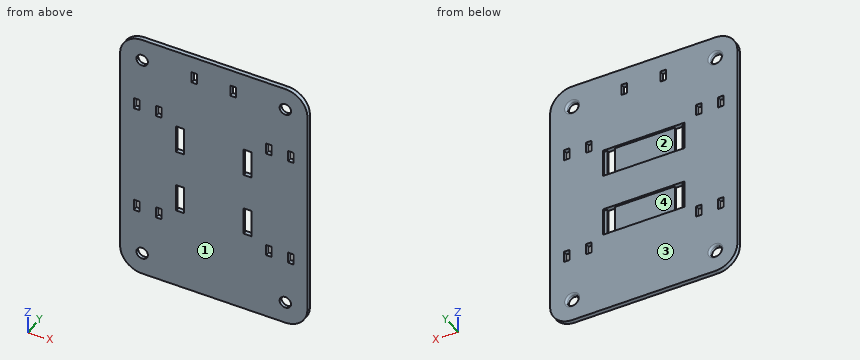
```python
from build123d import *

# Parameters (mm, degrees)
SKETCH1_W           = 107.95
SKETCH1_H           = 146.05
BOSS_EXTRUDE1_DEPTH = 2.54
SKETCH2_R           = 3.302
CUT_EXTRUDE1_DEPTH  = 91.842736914
SKETCH3_W           = 4.445
SKETCH3_H           = 15.875
CUT_EXTRUDE2_DEPTH  = 91.842736914
FILLET1_R           = 12.7
SKETCH11_W          = 47.200058
SKETCH11_H          = 15.875
CUT_EXTRUDE9_DEPTH  = 1.27
FILLET2_R           = 1.016
SKETCH14_W          = 3.175
SKETCH14_H          = 6.35
CUT_EXTRUDE14_DEPTH = 91.842736914


with BuildPart() as part:
    # Sketch1 → Boss-Extrude1 (new body)
    with BuildSketch(Plane(origin=(0, 0, 0), x_dir=(1, 0, 0), z_dir=(0, 1, 0))):
        Rectangle(SKETCH1_W, SKETCH1_H)
    extrude(amount=-BOSS_EXTRUDE1_DEPTH)

    # Sketch2 → Cut-Extrude1 (cut, through all)
    with BuildSketch(Plane(origin=(0, 0, 0), x_dir=(1, 0, 0), z_dir=(0, 1, 0))):
        with Locations(Location((-41.275, 60.325, 0), (0, 0, 270))):
            Circle(SKETCH2_R)
        with Locations(Location((41.275, 60.325, 0), (0, 0, 90))):
            Circle(SKETCH2_R)
        with Locations(Location((41.275, -60.325, 0), (0, 0, 270))):
            Circle(SKETCH2_R)
        with Locations(Location((-41.275, -60.325, 0), (0, 0, 90))):
            Circle(SKETCH2_R)
    extrude(amount=-CUT_EXTRUDE1_DEPTH, mode=Mode.SUBTRACT)

    # Sketch3 → Cut-Extrude2 (cut, through all)
    with BuildSketch(Plane(origin=(0, 0, 0), x_dir=(1, 0, 0), z_dir=(0, 1, 0))):
        with Locations((-19.472529, 18.374995)):
            Rectangle(SKETCH3_W, SKETCH3_H)
        with Locations((19.472529, 18.374995)):
            Rectangle(SKETCH3_W, SKETCH3_H)
        with Locations((19.472529, -18.374995)):
            Rectangle(SKETCH3_W, SKETCH3_H)
        with Locations((-19.472529, -18.374995)):
            Rectangle(SKETCH3_W, SKETCH3_H)
    extrude(amount=-CUT_EXTRUDE2_DEPTH, mode=Mode.SUBTRACT)

    # Fillet1
    fillet1_edges = [part.edges().sort_by_distance(p)[0] for p in [
        (53.975, -1.27, 73.025),
        (-53.975, -1.27, 73.025),
        (-53.975, -1.27, -73.025),
        (53.975, -1.27, -73.025),
    ]]
    fillet(fillet1_edges, radius=FILLET1_R)

    # Sketch11 → Cut-Extrude9 (cut, symmetric)
    with BuildSketch(Plane(origin=(0, 0, 0), x_dir=(1, 0, 0), z_dir=(0, 1, 0))):
        with Locations((0, -18.374995)):
            Rectangle(SKETCH11_W, SKETCH11_H)
        with Locations((0, 18.374995)):
            Rectangle(SKETCH11_W, SKETCH11_H)
    extrude(amount=CUT_EXTRUDE9_DEPTH, both=True, mode=Mode.SUBTRACT)

    # Fillet2
    fillet2_edges = [part.edges().sort_by_distance(p)[0] for p in [
        (-41.275, 0, -63.627),
        (41.275, 0, -57.023),
        (41.275, 0, 57.023),
        (-41.275, 0, 63.627),
    ]]
    fillet(fillet2_edges, radius=FILLET2_R)

    # Sketch14 → Cut-Extrude14 (cut, through all)
    with BuildSketch(Plane(origin=(0, 0, 0), x_dir=(1, 0, 0), z_dir=(0, 1, 0))):
        with Locations((31.7373, -31.75)):
            Rectangle(SKETCH14_W, SKETCH14_H)
        with Locations((-31.7373, -31.75)):
            Rectangle(SKETCH14_W, SKETCH14_H)
        with Locations((-31.7373, 31.75)):
            Rectangle(SKETCH14_W, SKETCH14_H)
        with Locations((31.7373, 31.75)):
            Rectangle(SKETCH14_W, SKETCH14_H)
        with Locations((-11.1125, -60.325)):
            Rectangle(SKETCH14_W, SKETCH14_H)
        with Locations((11.1125, -60.325)):
            Rectangle(SKETCH14_W, SKETCH14_H)
        with Locations((44.4627, 31.75)):
            Rectangle(SKETCH14_W, SKETCH14_H)
        with Locations((44.4627, -31.75)):
            Rectangle(SKETCH14_W, SKETCH14_H)
        with Locations((-44.4627, 31.75)):
            Rectangle(SKETCH14_W, SKETCH14_H)
        with Locations((-44.4627, -31.75)):
            Rectangle(SKETCH14_W, SKETCH14_H)
    extrude(amount=-CUT_EXTRUDE14_DEPTH, mode=Mode.SUBTRACT)


solid = part.part
```
Geometry check sheet. Reference: the model listing, model coordinates, mm. Face numbers are marked on the shaded views. A direction names the side the tool comes from. Coordinates: 2 decimals unless noted, no trailing zeros. Loops run counter-clockwise (first coordinate to the right, second up) from the corner with the lowest first, then second, coordinate; pieces in that order, holes last. Notation, with made-up numbers: (21, 34.25) -> (75, 34.25) arc R5 cw to (75, 42.25) -> close; hole circle Ø8 at (27.25, -18.75). An arc over 180 degrees is marked (long way). Put each result on its own line as item: value.
1) Thickness scan on line 1 (Z direction, x = -7, y = -0.65) (1 decimal); line 2 (X direction, y = -1.4, z = -21) (3 decimals); line 3 (Z direction, x = -40.5, y = -0.6) (3 decimals). Record the ranges inside material, lowest first.
Result set:
line 1: z = -73 to -26.3, -10.4 to 10.4, 26.3 to 73
line 2: x = -53.975 to -21.695, -17.25 to 17.25, 21.695 to 53.975
line 3: z = -73.025 to -63.626, -57.024 to 57.024, 63.626 to 73.025
2) Release check for a two-part mould opening along X. For the marked faces 3 and 4 record: released by +X, released by -X, zero draft, split by the parting line, or undercut.
Result set:
face 3: zero draft
face 4: undercut
3) Tool access check on the marked faces 1 and 2. Record the directions out of +Z, -Z, +X, -X, +Y, -Y that give a thin tool (end or side, any length) a straight path to the whole face; none if there is none.
Result set:
face 1: +Z, -Z, +X, -X, -Y
face 2: +Y
4) Gauge pin test, flat ends, axial feed: pin 1 Ø1.3 at (x, y) = (45, -1.5) entering from +Z; pin 2 Ø5 at (x, z) = (12, -10.5) entering from +Y; pin 3 Ø0.8 at (x, y) = (-45, -2) entering from -Z; pin 4 Ø1 at (x, z) = (22.5, 15.5) entering from +Y. Record the tip position at first contact, or that the pin passes through.
Result set:
pin 1: stops at z = 72.65
pin 2: stops at y = 0
pin 3: stops at z = -72.58
pin 4: stops at y = -1.27
5) Cross-section at A-A on z = -32.5. Record the boundary of the cut face in (x, y) (3 decimals), plus the area to 3 significant figures.
Result set:
outline: (-53.975, -2.54) -> (-46.05, -2.54) -> (-46.05, 0) -> (-53.975, 0) -> close; (-42.875, -2.54) -> (-33.325, -2.54) -> (-33.325, 0) -> (-42.875, 0) -> close; (-30.15, -2.54) -> (30.15, -2.54) -> (30.15, 0) -> (-30.15, 0) -> close; (33.325, -2.54) -> (42.875, -2.54) -> (42.875, 0) -> (33.325, 0) -> close; (46.05, -2.54) -> (53.975, -2.54) -> (53.975, 0) -> (46.05, 0) -> close
area: 242 mm^2
6) Cross-section at B-B on y = -1.85. Count the separate pieces of the cut face and the enclosed holes in it, plus the area to 3 significant figures.
Result set:
separate pieces: 1
enclosed holes: 18
area: 15,000 mm^2
